from build123d import *

# Parameters (mm, degrees)
RESSALTO_EXTRUS_O1_DEPTH      = 5
RESSALTO_EXTRUS_O1_DEPTH_BACK = 3.5
ESBO_O1_3_W                   = 105
ESBO_O1_3_H                   = 12.85
ESBO_O1_3_W_2                 = 21
ESBO_O1_3_H_2                 = 7.5
RESSALTO_EXTRUS_O2_DEPTH      = 3.5
ESBO_O1_4_W                   = 105
ESBO_O1_4_H                   = 12.85
ESBO_O1_4_W_2                 = 21
ESBO_O1_4_H_2                 = 7.5
RESSALTO_EXTRUS_O3_DEPTH      = 1
ESBO_O2_R                     = 1.3
CORTE_EXTRUS_O2_DEPTH         = 16.85


with BuildPart() as part:
    # Esbo_o1 → Ressalto-extrus_o1 (new body, two sides)
    with BuildSketch(Plane.XY) as ressalto_extrus_o1_sk:
        Polygon((-106, 18.391143911), (-95, 18.391143911), (2, 18.391143911), (2, 2.541143911), (-93, 2.541143911), (-106, 2.541143911), align=None)
        Polygon((-104.5, 16.891143911), (-104.5, 4.041143911), (-94.5, 4.041143911), (0.5, 4.041143911), (0.5, 16.891143911), (-96.5, 16.891143911), align=None, mode=Mode.SUBTRACT)
    extrude(amount=RESSALTO_EXTRUS_O1_DEPTH)
    extrude(ressalto_extrus_o1_sk.sketch, amount=-RESSALTO_EXTRUS_O1_DEPTH_BACK)

    # Esbo_o1_3 → Ressalto-extrus_o2 (add)
    with BuildSketch(Plane.XY):
        with Locations((-52, 10.466143911)):
            Rectangle(ESBO_O1_3_W, ESBO_O1_3_H)
        with Locations((-91.5, 10.641143911)):
            Rectangle(ESBO_O1_3_W_2, ESBO_O1_3_H_2, mode=Mode.SUBTRACT)
    extrude(amount=-RESSALTO_EXTRUS_O2_DEPTH)

    # Esbo_o1_4 → Ressalto-extrus_o3 (add)
    with BuildSketch(Plane.XY):
        with Locations((-52, 10.466143911)):
            Rectangle(ESBO_O1_4_W, ESBO_O1_4_H)
        with Locations((-91.5, 10.641143911)):
            Rectangle(ESBO_O1_4_W_2, ESBO_O1_4_H_2, mode=Mode.SUBTRACT)
    extrude(amount=RESSALTO_EXTRUS_O3_DEPTH)

    # Esbo_o2 → Corte-extrus_o2 (cut, through all)
    with BuildSketch(Plane(origin=(0, 18.391143911, -18.391143911), x_dir=(1, 0, 0), z_dir=(0, -1, 0))):
        with Locations((-96.75, 16.891143911)):
            Circle(ESBO_O2_R)
        with Locations((-87.25, 16.891143911)):
            Circle(ESBO_O2_R)
    extrude(amount=CORTE_EXTRUS_O2_DEPTH, mode=Mode.SUBTRACT)


solid = part.part
Source: CAD feature listing. Evaluate the final solid. Frame: model axes, mm. A direction names the side the tool comes from. Coordinates: 2 decimals unless noted, no trailing zeros. Order: outer loops, then holes, each group sorted by start corner. A loop starts at its lowest first (then second) coordinate and runs counter-clockwise, first axis right, second up.
Item 1: Cut plane D-D (x = -40). Return loops of the section in (y, z).
Output values:
outline: (2.54, -3.5) - (18.39, -3.5) - (18.39, 5) - (16.89, 5) - (16.89, 1) - (4.04, 1) - (4.04, 5) - (2.54, 5) - close
Item 2: Material intervals for line 1 (X direction, y = 17.5, z = -1.5); line 2 (X direction, y = 9.75, z = 3); line 3 (Y direction, x = -51.5, z = 2.5), sorted ascending.
Output values:
line 1: x = -106 to -98.05, -95.45 to -88.55, -85.95 to 2
line 2: x = -106 to -104.5, 0.5 to 2
line 3: y = 2.54 to 4.04, 16.89 to 18.39
Item 3: Cut plane A-A (z = -1.5). Return loops of the section in (x, y).
Output values:
outline: (-106, 2.54) - (-98.05, 2.54) - (-98.05, 6.89) - (-102, 6.89) - (-102, 14.39) - (-98.05, 14.39) - (-98.05, 18.39) - (-106, 18.39) - close; (-95.45, 2.54) - (-88.55, 2.54) - (-88.55, 6.89) - (-95.45, 6.89) - close; (-95.45, 14.39) - (-88.55, 14.39) - (-88.55, 18.39) - (-95.45, 18.39) - close; (-85.95, 2.54) - (2, 2.54) - (2, 18.39) - (-85.95, 18.39) - (-85.95, 14.39) - (-81, 14.39) - (-81, 6.89) - (-85.95, 6.89) - close
Item 4: First-contact query: P1, Ø4, axis at x = -44, y = 12, coming from the +Z side. Flat tip, straight axial feed; report the tip coordinate or a pass-through.
Output values:
P1: stops at z = 1
Item 5: Cut plane C-C (y = 11.5). Return loops of the section in (x, z).
Output values:
outline: (-106, -3.5) - (-102, -3.5) - (-102, 1) - (-104.5, 1) - (-104.5, 5) - (-106, 5) - close; (-81, -3.5) - (2, -3.5) - (2, 5) - (0.5, 5) - (0.5, 1) - (-81, 1) - close
Item 6: Cut plane B-B (x = -93). Return loops of the section in (y, z).
Output values:
outline: (2.54, -3.5) - (6.89, -3.5) - (6.89, 1) - (4.04, 1) - (4.04, 5) - (2.54, 5) - close; (14.39, -3.5) - (18.39, -3.5) - (18.39, 5) - (16.89, 5) - (16.89, 1) - (14.39, 1) - close
Item 7: Pull-direction query (Y, two-part tool) for faces 4 (the face through (-95.55, 4.75, -2)), 5 (the face through (-92, 14.391, -1)), 6 (the face through (-51, 18.391, 1)); classes: pulls with the +Y half, pulls with the -Y half, needs draft (parallel to the pull), parting line crosses it, or undercut.
Output values:
face 4: needs draft
face 5: undercut
face 6: pulls with the +Y half
Item 8: Set-up query: faces 1 (the face through (-81, 11, -1)), 2 (the face through (-53, 11, -3.5)), 3 (the face through (-104.5, 11, 3)). Return all of +Z, -Z, +X, -X, +Y, -Y with unobstructed straight access to the full face (end or side cutting, diameter ignored); none if empty.
Output values:
face 1: +Z, -Z
face 2: -Z, +X, -X, +Y, -Y
face 3: +Z
